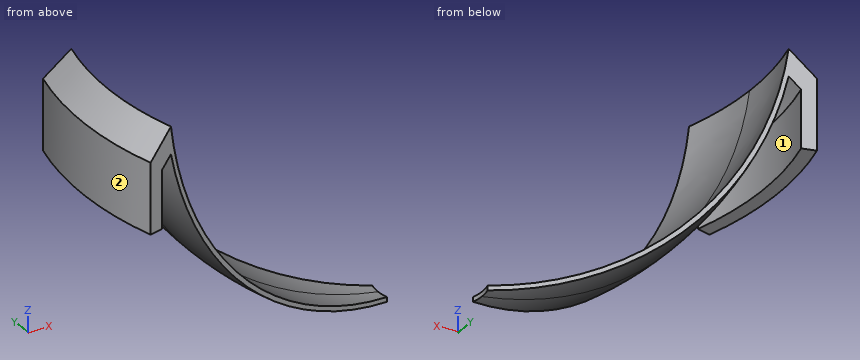
from build123d import *

# Parameters (mm, degrees)
F1_ANGLE = 30


with BuildPart() as f1:
    # F0 (on Front) → F1 (revolve, symmetric)
    with BuildSketch(Plane.XZ) as f1_sk:
        with BuildLine():
            ThreePointArc((32.006004, -22.18296), (12.573001, -12.326296), (3, 7.248))
            Line((3, 7.248), (0.271143, 4.519142))
            Line((0.271143, 4.519142), (0.271143, -3.053563))
            Line((0.271143, -3.053563), (1.601774, -3.053563))
            Line((1.601774, -3.053563), (1.804178, -3.053563))
            Line((1.804178, -3.053563), (1.804178, 3.149904))
            Line((1.804178, 3.149904), (3, 4.345534))
            ThreePointArc((3, 4.345534), (13.27576, -13.706999), (32.006004, -22.688268))
            Line((32.006004, -22.688268), (32.006004, -22.18296))
        make_face()
    revolve(axis=Axis((37, 0, -38.976204), (0, 0, 1)), revolution_arc=F1_ANGLE / 2)
    revolve(f1_sk.sketch, axis=Axis((37, 0, -38.976204), (0, 0, -1)), revolution_arc=F1_ANGLE / 2)


solid = f1.part
Geometry check sheet. Reference: the model listing, model coordinates, mm. Face numbers are marked on the shaded views. A direction names the side the tool comes from. Give positions to 0.01 mm unless a question says otherwise; leave off trailing zeros. Use one line per item in the form item = value.
1) Depth check by flat-ended pin: pin 1 Ø2 at (x, y) = (1, -1.5) entering from -Z; pin 2 Ø1 at (x, y) = (9.5, 5) entering from -Z; pin 3 Ø6 at (x, y) = (5, 7) entering from -Z. Enter the tip coordinate at first touch or a pass-through.
Working result:
pin_1 = -3.05
pin_2 = -9.64
pin_3 = -6.29
2) Material ranges on probe 1 along X at (y, z) = (-6.5, -1.5); probe 2 along X at (y, z) = (-7.25, -1.5); probe 3 along X at (y, z) = (-1.5, -8.25), recorded low to high. Write a range as from..to.
Working result:
probe_1 = 0.85..2.41, 5.49..6.04
probe_2 = 0.99..2.56, 5.65..6.21
probe_3 = 8.56..9.18
3) Access from +Z, -Z, +X, -X, +Y, -Y to the whole of each face (thin tool, end or side, straight path). Record for the marked faces 1 and 2.
Working result:
face_1 = -Z
face_2 = +Z, -Z, -X
